Work out the finished part from the listing and answer in its coordinate system (mm). A direction names the side the tool comes from. Round coordinates to 2 decimals unless told otherwise and drop trailing zeros. Order: outer loops, then holes, each group sorted by start corner. A loop starts at its lowest first (then second) coordinate and runs counter-clockwise, first axis right, second up. Notation, with made-up numbers: (17.5, 60) - (45.5, 60) arc R26 ccw to (45.5, 78) - close; hole circle Ø2 at (-39, -5.5). An arc over 180 degrees is marked (long way). Answer in a Markdown table with one row per item.
from build123d import *

# Parameters (mm, degrees)
F0_W     = 600
F0_H     = 600
F0_W_2   = 596
F0_H_2   = 596
F1_DEPTH = 179
F2_R     = 7.5
F3_DEPTH = 25
F4_R     = 7.5
F5_DEPTH = 25


with BuildPart() as f1:
    # F0 (on Right) → F1 (new body)
    with BuildSketch(Plane.YZ):
        with Locations((107.142857, 0.014796)):
            Rectangle(F0_W, F0_H)
        with Locations((107.142857, 0.014796)):
            Rectangle(F0_W_2, F0_H_2, mode=Mode.SUBTRACT)
    extrude(amount=F1_DEPTH)

    # F2 (on face) → F3 (cut)
    with BuildSketch(Plane.XY.offset(300.014796)):
        with Locations((25, -145.957143)):
            Circle(F2_R)
        with Locations((80.5, -3.957143)):
            Circle(F2_R)
        with Locations((125.5, -3.957143)):
            Circle(F2_R)
        with Locations((125.5, -104.857143)):
            Circle(F2_R)
    extrude(amount=-F3_DEPTH, mode=Mode.SUBTRACT)

    # F4 (on face) → F5 (cut)
    with BuildSketch(Plane.XZ.offset(192.857143)):
        with Locations((80.5, -191.285204)):
            Circle(F4_R)
    extrude(amount=-F5_DEPTH, mode=Mode.SUBTRACT)


solid = f1.part
1) Find section C-C, the plane x = 109.5. Give the vertices of the cut face in (y, z).
Filled in:
| item | result |
|---|---|
| outline | (-192.86, -299.99) - (407.14, -299.99) - (407.14, 300.01) - (-192.86, 300.01) - close; hole (-190.86, -297.99) - (405.14, -297.99) - (405.14, 298.01) - (-190.86, 298.01) - close |
2) Find the intervals of material crossed by probe 1 along Y at (x, z) = (125.5, 298.85); probe 2 along Z at (x, y) = (93.5, -57.5); probe 3 along Y at (x, z) = (139.5, -201.5), in increasing order. Write a range as from..to.
Filled in:
| item | result |
|---|---|
| probe 1 | y = -192.86..-112.36, -97.36..-11.46, 3.54..407.14 |
| probe 2 | z = -299.99..-297.99, 298.01..300.01 |
| probe 3 | y = -192.86..-190.86, 405.14..407.14 |
3) The mould has two halves that part along Y. Classify faces 4 (the face through (88, 103, 300.015)), 5 (the face through (132.43, -6.83, 299.03)), 6 (the face through (88, 407.143, -4)): released by +Y, released by -Y, zero draft, split by the parting line, or undercut.
Filled in:
| item | result |
|---|---|
| face 4 | zero draft |
| face 5 | undercut |
| face 6 | released by +Y |
4) Find section D-D, the plane x = 25. Give the vertices of the cut face in (y, z).
Filled in:
| item | result |
|---|---|
| outline | (-192.86, -299.99) - (407.14, -299.99) - (407.14, 300.01) - (-138.46, 300.01) - (-138.46, 298.01) - (405.14, 298.01) - (405.14, -297.99) - (-190.86, -297.99) - (-190.86, 298.01) - (-153.46, 298.01) - (-153.46, 300.01) - (-192.86, 300.01) - close |
5) Find section B-B, the plane z = 212. Give the vertices of the cut face in (x, y).
Filled in:
| item | result |
|---|---|
| outline | (0, -192.86) - (179, -192.86) - (179, -190.86) - (0, -190.86) - close; (0, 405.14) - (179, 405.14) - (179, 407.14) - (0, 407.14) - close |
6) Find section A-A, the plane y = 267. Give the vertices of the cut face in (x, z), then the cut area to 3 significant figures.
Filled in:
| item | result |
|---|---|
| outline | (0, -299.99) - (179, -299.99) - (179, -297.99) - (0, -297.99) - close; (0, 298.01) - (179, 298.01) - (179, 300.01) - (0, 300.01) - close |
| area | 716 mm^2 |
7) Which of the six approach directions +Z, -Z, +X, -X, +Y, -Y give full straight-line access (tool end or side, diameter ignored) to faces 1 (the face through (74.55, -191.87, -195.85)), 2 (the face through (88, 103, 298.015)), 3 (the face through (73, -4, 299))?
Filled in:
| item | result |
|---|---|
| face 1 | -Y |
| face 2 | +X, -X |
| face 3 | +Z |
8) Each of these flat-tipped pins is pushed along its axis until it touches: pin 1 (13.5 mm diameter, centred on x = 125.5, y = -104.86, fed in from +Z); pin 2 (9 mm diameter, centred on x = 80.5, z = -191.29, fed in from -Y). Where does it stop, or does it pass through?
Filled in:
| item | result |
|---|---|
| pin 1 | stops at z = -297.99 |
| pin 2 | stops at y = 405.14 |
